Check sheet for the modelled part. Datum: model origin and axes. Units: mm. Round coordinates to 2 decimals unless told otherwise and drop trailing zeros. Loops run counter-clockwise (first coordinate to the right, second up) from the corner with the lowest first, then second, coordinate; pieces in that order, holes last. Notation, with made-up numbers: (-31.5, 4) -> (-24.5, 4) arc R28 cw to (-24.5, 32) -> close; hole circle Ø9 at (11, -8). An arc over 180 degrees is marked (long way). Return JSON: item names as keys, results as strings.
from build123d import *

# Parameters (mm, degrees)
F0_W        = 130
F0_H        = 75
F1_DEPTH    = 3
F2_T1_DEPTH = 153.1732604525
F2_T3_DEPTH = 98.1732604525
F4_W        = 129.1797161102
F4_H        = 75.0736519694
F5_DEPTH    = 3


# Not quite as in the source:
# - a fillet or chamfer that OpenCascade refuses, or shapes differently, is made with other operations: its cross-section is extruded or revolved along the edge and cut away or added


with BuildPart() as f1:
    # F0 (on Top) → F1 (new body)
    with BuildSketch(Plane.XY):
        Rectangle(F0_W, F0_H)
    extrude(amount=F1_DEPTH)

    # F2: fillet of radius 5.08 on 4 edges, made by hand

    # F2_s2 → F2_t1 (cut)
    with BuildSketch(Plane.YZ.offset(-76.5866302263)):
        with BuildLine():
            ThreePointArc((37.5, 3), (35.6257826579, 0.8154484409), (32.8653479095, 0))
            Line((32.8653479095, 0), (37.5, 0))
            Line((37.5, 0), (37.5, 3))
        make_face()
        with BuildLine():
            ThreePointArc((-37.5, 3), (-35.6257826579, 0.8154484409), (-32.8653479095, 0))
            Line((-32.8653479095, 0), (-37.5, 0))
            Line((-37.5, 0), (-37.5, 3))
        make_face()
    extrude(amount=F2_T1_DEPTH, mode=Mode.SUBTRACT)

    # F2_s4 → F2_t3 (cut)
    with BuildSketch(Plane.XZ.offset(-49.0866302263)):
        with BuildLine():
            ThreePointArc((65, 3), (63.1257826579, 0.8154484409), (60.3653479095, 0))
            Line((60.3653479095, 0), (65, 0))
            Line((65, 0), (65, 3))
        make_face()
        with BuildLine():
            ThreePointArc((-65, 3), (-63.1257826579, 0.8154484409), (-60.3653479095, 0))
            Line((-60.3653479095, 0), (-65, 0))
            Line((-65, 0), (-65, 3))
        make_face()
    extrude(amount=F2_T3_DEPTH, mode=Mode.SUBTRACT)

    # F4 (on face) → F5 (join)
    with BuildSketch(Plane.XY.offset(3)):
        Rectangle(F4_W, F4_H)
    extrude(amount=F5_DEPTH)


solid = f1.part
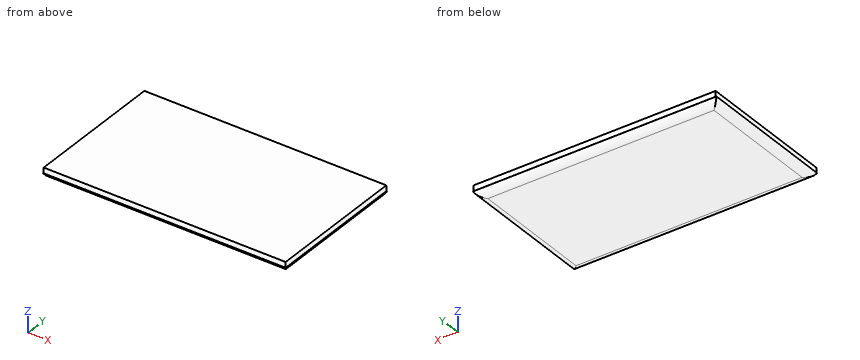
Q1. Section check B-B (z = 1.15). Record the boundary of the cut face in (x, y), then the cut area to 3 significant figures.
Results list:
{"outline": "(-63.58, -36.08) -> (63.58, -36.08) -> (63.58, 36.08) -> (-63.58, 36.08) -> close", "area": "9,180 mm^2"}
Q2. Go/stop test with flat-tipped pins: pin 1 (1.5 mm diameter, centred on x = -51.5, z = 2, fed in from +Y); pin 2 (3.5 mm diameter, centred on y = 2.5, z = 5, fed in from +X). Record where each tip stops, or that it passes through.
Results list:
{"pin 1": "y = 37.38", "pin 2": "x = 64.59"}
Q3. Material ranges on line 1 (X direction, y = 13, z = 5.45); line 2 (X direction, y = -1.5, z = 1.15); line 3 (Y direction, x = -18.5, z = 1.5), recorded low to high.
Results list:
{"line 1": "-64.59 to 64.59", "line 2": "-63.58 to 63.58", "line 3": "-36.47 to 36.47"}
